Geometry check sheet. Reference: the model listing, model coordinates, mm. Face numbers are marked on the shaded views. Give positions to 0.01 mm unless a question says otherwise; leave off trailing zeros. Write each loop counter-clockwise with the first axis right and the second up, starting at its lowest first coordinate (ties: lowest second). Pieces come first, ordered by that corner, then holes. Notation, with made-up numbers: (55, 50) - (81, 50) arc R23 cw to (81, 79) - close; hole circle Ø10 at (-20.75, 20). An arc over 180 degrees is marked (long way). Use a Markdown table: item, result.
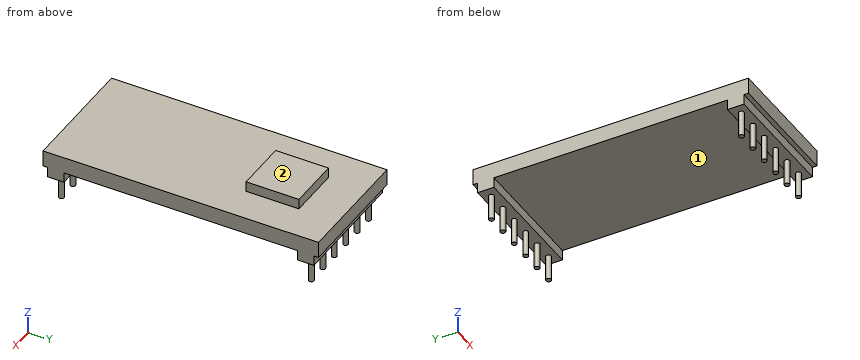
```python
from build123d import *

# Parameters (mm, degrees)
F0_W     = 12
F0_H     = 27
F1_DEPTH = 1.6
F2_W     = 12
F2_H     = 1.6
F3_DEPTH = 1
F4_R     = 0.25
F5_DEPTH = 2.5
F6_W     = 5.18181
F6_H     = 5.181811
F7_DEPTH = 1


with BuildPart() as f1:
    # F0 (on Top) → F1 (new body)
    with BuildSketch(Plane.XY):
        Rectangle(F0_W, F0_H)
    extrude(amount=F1_DEPTH)

    # F2 (on face) → F3 (join)
    with BuildSketch(Plane(origin=(0, 0, 0), x_dir=(1, 0, 0), z_dir=(0, 0, -1))):
        with Locations((0, -12.25)):
            Rectangle(F2_W, F2_H)
        with Locations((0, 12.25)):
            Rectangle(F2_W, F2_H)
    extrude(amount=F3_DEPTH)

    # F4 (on face) → F5 (join)
    with BuildSketch(Plane(origin=(0, 0, -1), x_dir=(1, 0, 0), z_dir=(0, 0, -1))):
        with Locations((-5, -12.25)):
            Circle(F4_R)
        with Locations((-5, 12.25)):
            Circle(F4_R)
        with Locations((-3, -12.25)):
            Circle(F4_R)
        with Locations((-3, 12.25)):
            Circle(F4_R)
        with Locations((-1, -12.25)):
            Circle(F4_R)
        with Locations((-1, 12.25)):
            Circle(F4_R)
        with Locations((1, -12.25)):
            Circle(F4_R)
        with Locations((1, 12.25)):
            Circle(F4_R)
        with Locations((3, -12.25)):
            Circle(F4_R)
        with Locations((3, 12.25)):
            Circle(F4_R)
        with Locations((5, -12.25)):
            Circle(F4_R)
        with Locations((5, 12.25)):
            Circle(F4_R)
    extrude(amount=F5_DEPTH)

    # F6 (on face) → F7 (join)
    with BuildSketch(Plane.XY.offset(1.6)):
        with Locations((0, 7.086888)):
            Rectangle(F6_W, F6_H)
    extrude(amount=F7_DEPTH)


solid = f1.part
```
1) Material ranges on L1, parallel to Y at x = -4.25, z = -0.25; L2, parallel to Z at x = 1.5, y = 7.75; L3, parallel to Y at x = -3, z = -1.5, recorded low to high. Write a range as from..to.
Working result:
| item | result |
|---|---|
| L1 | y = -13.05..-11.45, 11.45..13.05 |
| L2 | z = 0..2.6 |
| L3 | y = -12.5..-12, 12..12.5 |
2) Section check A-A on z = -1.75. Count the separate pieces of the cut face and the enclosed holes in it, then the cut area to 3 significant figures.
Working result:
| item | result |
|---|---|
| separate pieces | 12 |
| enclosed holes | 0 |
| area | 2.36 mm² |
3) Depth check by flat-ended pin: P1, Ø5, axis at x = 2, y = -7, coming from the +Z side; P2, Ø0.5, axis at x = -2, y = -13.5, coming from the -Z side; P3, Ø0.5, axis at x = 1, z = 2, coming from the -Y side. Enter the tip coordinate at first touch or a pass-through.
Working result:
| item | result |
|---|---|
| P1 | stops at z = 1.6 |
| P2 | stops at z = 0 |
| P3 | stops at y = 4.5 |
4) Mould release check, pull along Y, two halves, no side actions. Record for the marked faces 1 and 2: pulls with the +Y half, pulls with the -Y half, needs draft (parallel to the pull), parting line crosses it, or undercut.
Working result:
| item | result |
|---|---|
| face 1 | undercut |
| face 2 | needs draft |
5) Section check C-C on y = -12.25. Record the boundary of the cut face in (x, z), then the cut area to 3 significant figures.
Working result:
| item | result |
|---|---|
| outline | (-6, -1) - (-5.25, -1) - (-5.25, -3.5) - (-4.75, -3.5) - (-4.75, -1) - (-3.25, -1) - (-3.25, -3.5) - (-2.75, -3.5) - (-2.75, -1) - (-1.25, -1) - (-1.25, -3.5) - (-0.75, -3.5) - (-0.75, -1) - (0.75, -1) - (0.75, -3.5) - (1.25, -3.5) - (1.25, -1) - (2.75, -1) - (2.75, -3.5) - (3.25, -3.5) - (3.25, -1) - (4.75, -1) - (4.75, -3.5) - (5.25, -3.5) - (5.25, -1) - (6, -1) - (6, 1.6) - (-6, 1.6) - close |
| area | 38.7 mm² |
6) Section check D-D on x = 4. Record the boundary of the cut face in (y, z), then the cut area to 3 significant figures.
Working result:
| item | result |
|---|---|
| outline | (-13.5, 0) - (-13.05, 0) - (-13.05, -1) - (-11.45, -1) - (-11.45, 0) - (11.45, 0) - (11.45, -1) - (13.05, -1) - (13.05, 0) - (13.5, 0) - (13.5, 1.6) - (-13.5, 1.6) - close |
| area | 46.4 mm² |
7) Section check B-B on x = 0. Record the boundary of the cut face in (y, z).
Working result:
| item | result |
|---|---|
| outline | (-13.5, 0) - (-13.05, 0) - (-13.05, -1) - (-11.45, -1) - (-11.45, 0) - (11.45, 0) - (11.45, -1) - (13.05, -1) - (13.05, 0) - (13.5, 0) - (13.5, 1.6) - (9.68, 1.6) - (9.68, 2.6) - (4.5, 2.6) - (4.5, 1.6) - (-13.5, 1.6) - close |
